Autodesk Inventor part; units mm, degrees
ref_plane "YZ Plane" through (0, 0, 0) normal (1, 0, 0) x (0, 1, 0)
ref_plane "XZ Plane" through (0, 0, 0) normal (0, 1, 0) x (-1, 0, 0)
ref_plane "XY Plane" through (0, 0, 0) normal (0, 0, 1) x (1, 0, 0)
sketch "Sketch2" plane through (0, 0, 0) normal (0, 0, 1) x (1, 0, 0)
  line L0 (87, 75) -> (-87, 75)
  line L1 (-87, 75) -> (-87, -75)
  line L2 (-87, -75) -> (87, -75)
  line L3 (87, -75) -> (87, 75)
  line L4 (87, 75) -> (-87, -75) construction
  line L5 (-87, 75) -> (87, -75) construction
  point P0 (0, 0)
  dimension "d3" = 174
  dimension "d4" = 150
sketch "Sketch1" plane through (0, 0, 0) normal (0, 0, 1) x (1, 0, 0)
  line L0 (77, 56) -> (-77, 56)
  line L1 (-77, 56) -> (-77, -56)
  line L2 (-77, -56) -> (77, -56)
  line L3 (77, -56) -> (77, 56)
  line L4 (77, 56) -> (-77, -56) construction
  line L5 (-77, 56) -> (77, -56) construction
  arc A0 (77, 3.5816) -> (24.5816, 56) centre (24.5816, 3.5816) ccw
  line L6 (-77, -56) -> (59.13, 43.0036) construction
  arc A1 (-24.5816, 56) -> (-77, 3.5816) centre (-24.5816, 3.5816) ccw
  point P0 (0, 0)
  dimension "d0" = 154
  dimension "d1" = 112
  dimension "d2" = 136.13
extrude "Extrusion1" add sketch "Sketch2" against normal blind 200
extrude "Extrusion2" cut sketch "Sketch1" against normal blind 150 contours A0 L3 L2 L1 A1 L0
properties part number "thermostatBath"
Source: CAD feature listing. Evaluate the final solid. Frame: model axes, mm. A direction names the side the tool comes from. Coordinates: 2 decimals unless noted, no trailing zeros. Order: outer loops, then holes, each group sorted by start corner. A loop starts at its lowest first (then second) coordinate and runs counter-clockwise, first axis right, second up. Notation, with made-up numbers: (29.5, 15.25) - (39.5, 15.25) arc R25 ccw to (39.5, 39.25) - close; hole circle Ø10 at (-22, 77). An arc over 180 degrees is marked (long way). One line per item, written item: value.
1) Cut plane B-B on z = -37. Output: boundary loops of the cut face in (x, y).
Computed values:
outline: (-87, -75) - (87, -75) - (87, 75) - (-87, 75) - close; hole (-77, -56) - (77, -56) - (77, 3.58) arc R52.42 ccw to (24.58, 56) - (-24.58, 56) arc R52.42 ccw to (-77, 3.58) - close
2) Cut plane A-A on x = 6. Output: boundary loops of the cut face in (y, z), plus the area to 3 significant figures.
Computed values:
outline: (-75, -200) - (75, -200) - (75, 0) - (56, 0) - (56, -150) - (-56, -150) - (-56, 0) - (-75, 0) - close
area: 13,200 mm^2
3) Reachability of faces 5 (the face through (-1, 1, -200)), 6 (the face through (-61.24, 41.05, -73.95)) from +Z, -Z, +X, -X, +Y, -Y: full face, straight path, thin tool, end or side. Return the list, or none.
Computed values:
face 5: -Z, +X, -X, +Y, -Y
face 6: +Z
4) Contact query for a flat-ended pin moving along its axis: pin 1 (6 mm diameter, centred on x = 50, y = -50, fed in from +Z). Output: stop coordinate, or through.
Computed values:
pin 1: stops at z = -150
5) Ray query, line 1 (X direction, y = -11, z = -130); line 2 (Y direction, x = 17.5, z = -127); line 3 (Z direction, x = -26.5, y = 15). Return the intervals inside material, ascending. Write a range as [from, to].
Computed values:
line 1: x = [-87, -77], [77, 87]
line 2: y = [-75, -56], [56, 75]
line 3: z = [-200, -150]
6) Mould query, pull axis Y, two halves, no side actions, for faces 1 (the face through (0, 56, -74)), 2 (the face through (87, -1, -99)), 3 (the face through (1, 75, -99)), 4 (the face through (-1, -56, -74)). Classes: released by +Y, released by -Y, zero draft, split by the parting line, or undercut.
Computed values:
face 1: undercut
face 2: zero draft
face 3: released by +Y
face 4: undercut
7) Cut plane C-C on y = -8. Output: boundary loops of the cut face in (x, z).
Computed values:
outline: (-87, -200) - (87, -200) - (87, 0) - (77, 0) - (77, -150) - (-77, -150) - (-77, 0) - (-87, 0) - close
